```python
from build123d import *

# Parameters (mm, degrees)
SKETCH1_R           = 55
BOSS_EXTRUDE1_DEPTH = 20
SKETCH2_R           = 70
BOSS_EXTRUDE2_DEPTH = 20
SKETCH3_R           = 40
BOSS_EXTRUDE3_DEPTH = 60
CUT_EXTRUDE1_REACH  = 102
SKETCH4_R           = 30
BOSS_EXTRUDE4_REACH = 252
SKETCH6_W           = 80
SKETCH6_H           = 20
CUT_EXTRUDE2_DEPTH  = 60
BOSS_EXTRUDE5_REACH = 292
SKETCH10_W          = 40
SKETCH10_H          = 40
CUT_EXTRUDE3_DEPTH  = 60
SKETCH12_R          = 12.5
CUT_EXTRUDE4_DEPTH  = 60


with BuildPart() as part:
    # Sketch1 → Boss-Extrude1 (new body)
    with BuildSketch(Plane(origin=(0, 0, 0), x_dir=(1, 0, 0), z_dir=(0, 1, 0))):
        Circle(SKETCH1_R)
    extrude(amount=BOSS_EXTRUDE1_DEPTH)

    # Sketch2 → Boss-Extrude2 (add)
    with BuildSketch(Plane(origin=(0, 20, 0), x_dir=(1, 0, 0), z_dir=(0, 1, 0))):
        Circle(SKETCH2_R)
    extrude(amount=BOSS_EXTRUDE2_DEPTH)

    # Sketch3 → Boss-Extrude3 (add)
    with BuildSketch(Plane.XZ):
        Circle(SKETCH3_R)
    extrude(amount=BOSS_EXTRUDE3_DEPTH)

    # Sketch4 → Cut-Extrude1 (cut, up to next)
    with BuildSketch(Plane(origin=(0, 40, 0), x_dir=(1, 0, 0), z_dir=(0, 1, 0)), mode=Mode.PRIVATE) as cut_extrude1_sk1:
        Circle(SKETCH4_R)
    cut_extrude1_tool1 = extrude(cut_extrude1_sk1.sketch, amount=-CUT_EXTRUDE1_REACH, mode=Mode.PRIVATE) & part.part
    add(cut_extrude1_tool1.solids().sort_by_distance((0, 40, 0))[0], mode=Mode.SUBTRACT)

    # Sketch6 → Boss-Extrude4 (add, up to next)
    with BuildSketch(Plane(origin=(180, 0, 0), x_dir=(0, 0, -1), z_dir=(1, 0, 0)), mode=Mode.PRIVATE) as boss_extrude4_sk1:
        with Locations((0, -50)):
            Rectangle(SKETCH6_W, SKETCH6_H)
    boss_extrude4_tool1 = extrude(boss_extrude4_sk1.sketch, amount=-BOSS_EXTRUDE4_REACH, mode=Mode.PRIVATE) - part.part
    add(boss_extrude4_tool1.solids().sort_by_distance((180, -50, 0))[0])

    # Sketch8 → Cut-Extrude2 (cut)
    with BuildSketch(Plane(origin=(0, -40, 0), x_dir=(1, 0, 0), z_dir=(0, 1, 0))):
        with BuildLine():
            Line((180, 15), (180, -15))
            Line((180, -15), (128.7735226, -15))
            ThreePointArc((128.7735226, -15), (113.7735226, 0), (128.7735226, 15))
            Line((128.7735226, 15), (180, 15))
        make_face()
    extrude(amount=-CUT_EXTRUDE2_DEPTH, mode=Mode.SUBTRACT)

    # Sketch10 → Boss-Extrude5 (add, up to next)
    with BuildSketch(Plane(origin=(-110, 0, 0), x_dir=(0, 0, -1), z_dir=(1, 0, 0)), mode=Mode.PRIVATE) as boss_extrude5_sk1:
        with Locations((0, -40)):
            Rectangle(SKETCH10_W, SKETCH10_H)
    boss_extrude5_tool1 = extrude(boss_extrude5_sk1.sketch, amount=BOSS_EXTRUDE5_REACH, mode=Mode.PRIVATE) - part.part
    add(boss_extrude5_tool1.solids().sort_by_distance((-110, -40, 0))[0])

    # Sketch11 → Cut-Extrude3 (cut)
    with BuildSketch(Plane.XY.offset(20)):
        with BuildLine():
            ThreePointArc((-110, -40), (-104.142135624, -25.857864376), (-90, -20))
            Line((-90, -20), (-110, -20))
            Line((-110, -20), (-110, -40))
        make_face()
        with BuildLine():
            ThreePointArc((-90, -60), (-104.142135624, -54.142135624), (-110, -40))
            Line((-110, -40), (-110, -60))
            Line((-110, -60), (-90, -60))
        make_face()
    extrude(amount=-CUT_EXTRUDE3_DEPTH, mode=Mode.SUBTRACT)

    # Sketch12 → Cut-Extrude4 (cut)
    with BuildSketch(Plane.XY.offset(20)):
        with Locations((-90, -40)):
            Circle(SKETCH12_R)
    extrude(amount=-CUT_EXTRUDE4_DEPTH, mode=Mode.SUBTRACT)


solid = part.part
```
Build history of the part. All positions in model axes, mm. A direction names the side the tool comes from. Give positions to 0.01 mm unless a question says otherwise; leave off trailing zeros. Order: outer loops, then holes, each group sorted by start corner. A loop starts at its lowest first (then second) coordinate and runs counter-clockwise, first axis right, second up. Notation, with made-up numbers: M -29.75,62.5 L -12.75,62.5 A36 cw -12.75,101.5 Z; hole C 82,-17.75 d4. An arc over 180 degrees is marked long. Return JSON: item names as keys, results as strings.
Q1. Flat gauge pins, fed straight in: pin 1 (10 mm diameter, centred on x = 127.5, y = -49.5, fed in from -Z); pin 2 (8 mm diameter, centred on y = -15, z = -22, fed in from +X); pin 3 (6 mm diameter, centred on x = 120, y = -46.5, fed in from +Z); pin 4 (20 mm diameter, centred on x = -76, z = -6, fed in from +Y). Where does each tip first touch, or does it go through?
Answer list:
{"pin 1": "stops at z = -40", "pin 2": "stops at x = 35.72", "pin 3": "stops at z = 40", "pin 4": "stops at y = 40"}
Q2. 3-axis set-ups, long thin cutter, end or side, ignore diameter. For faces 1 (the face through (-64, -40, 20)), 2 (the face through (154, -50, -15)), 3 (the face through (91, -50, -40)), 4 (the face through (-42, 20, 36)): which of +Z, -Z, +X, -X, +Y, -Y reach the whole face in a straight line?
Answer list:
{"face 1": "+Z, -X, -Y", "face 2": "+X, +Y, -Y", "face 3": "-Z, +X, -X, -Y", "face 4": "none"}
Q3. Band-saw the part on C-C (z = -50.5). Give the cut face in (x, y).
Answer list:
{"outline": "M -48.47,20 L -21.79,20 L -21.79,0 L 21.79,0 L 21.79,20 L 48.47,20 L 48.47,40 L -48.47,40 Z"}
Q4. Two-plate mould, pull along Y, no slides. Class faces 5 (the face through (47, -60, 1)), 6 (the face through (-11.923, 9.86, 53.692)), 7 (the face through (180, -50, 28)): pulls with the +Y half, pulls with the -Y half, needs draft (parallel to the pull), parting line crosses it, or undercut.
Answer list:
{"face 5": "pulls with the -Y half", "face 6": "undercut", "face 7": "needs draft"}
Q5. Band-saw the part on A-A (z = 0). Give the cut face in (x, y), then the cut area to 3 significant figures.
Answer list:
{"outline": "M -90,-60 L -30,-60 L -30,40 L -70,40 L -70,20 L -55,20 L -55,0 L -40,0 L -40,-20 L -90,-20 A20 ccw Z; M 30,-60 L 113.77,-60 L 113.77,-40 L 40,-40 L 40,0 L 55,0 L 55,20 L 70,20 L 70,40 L 30,40 Z; hole C -90,-40 d25", "area": "7,410 mm^2"}
Q6. Band-saw the part on D-D (y = -17). Give the cut face in (x, z).
Answer list:
{"outline": "C 0,0 d80; hole C 0,0 d60"}
Q7. Wall check: probe 1 along Y at (x, z) = (20.5, -39.5); probe 2 along X at (y, z) = (-8, 0); probe 3 along Y at (x, z) = (-90, -8). Give the ranges that are in metal, low to high. Write a range as from..to.
Answer list:
{"probe 1": "y = -60..-40, 0..40", "probe 2": "x = -40..-30, 30..40", "probe 3": "y = -60..-52.5, -27.5..-20"}
Q8. Band-saw the part on B-B (x = -11.5). Give the cut face in (y, z).
Answer list:
{"outline": "M -60,-38.31 L 0,-38.31 L 0,-53.78 L 20,-53.78 L 20,-69.05 L 40,-69.05 L 40,-27.71 L -60,-27.71 Z; M -60,27.71 L 40,27.71 L 40,69.05 L 20,69.05 L 20,53.78 L 0,53.78 L 0,38.31 L -60,38.31 Z"}
